from build123d import *

# Parameters (mm, degrees)
ESQUISSE1_R                  = 28
BOSS_EXTRU_1_DEPTH           = 3
ENL_V_MAT_EXTRU_1_DEPTH      = 40.711459303
ENL_V_MAT_EXTRU_1_DEPTH_BACK = 40.711459303
ESQUISSE2_R                  = 3
ESQUISSE3_R                  = 12.75
ESQUISSE3_R_2                = 10.25
BOSS_EXTRU_2_DEPTH           = 10
CHANFREIN1_SIZE              = 2


with BuildPart() as part:
    # Esquisse1 → Boss.-Extru.1 (new body)
    with BuildSketch(Plane.XY):
        Circle(ESQUISSE1_R)
    extrude(amount=BOSS_EXTRU_1_DEPTH)

    # Esquisse2 → Enlèv. mat.-Extru.1 (cut, two sides: drawn at the far end of the back side and taken through both)
    with BuildSketch(Plane.XY.offset(3).offset(-ENL_V_MAT_EXTRU_1_DEPTH_BACK)):
        Circle(ESQUISSE2_R)
    extrude(amount=ENL_V_MAT_EXTRU_1_DEPTH + ENL_V_MAT_EXTRU_1_DEPTH_BACK, mode=Mode.SUBTRACT)

    # Esquisse3 → Boss.-Extru.2 (add)
    with BuildSketch(Plane.XY.offset(3)):
        Circle(ESQUISSE3_R)
        Circle(ESQUISSE3_R_2, mode=Mode.SUBTRACT)
    extrude(amount=BOSS_EXTRU_2_DEPTH)

    # Chanfrein1
    chanfrein1_edges = [part.edges().sort_by_distance(p)[0] for p in [
        (-12.75, 0, 3),
    ]]
    chamfer(chanfrein1_edges, length=CHANFREIN1_SIZE)


solid = part.part
For this review, take the finished solid that the model builds, in its own axes (mm). A direction names the side the tool comes from. Round coordinates to 2 decimals unless told otherwise and drop trailing zeros. Order: outer loops, then holes, each group sorted by start corner. A loop starts at its lowest first (then second) coordinate and runs counter-clockwise, first axis right, second up. Notation, with made-up numbers: (-20.5, -30) -> (-0.5, -30) arc R10 ccw to (-0.5, -19) -> close; hole circle Ø8 at (38.25, -1.5). An arc over 180 degrees is marked (long way). Write item = value, one per line. Start each with the question number.
1) To check wall thickness, follow line 1 (Y direction, x = 0, z = 5.25); line 2 (Z direction, x = 20, y = -1); line 3 (Y direction, x = -5, z = 6). State the ranges of each line that lie inside material, in increasing order. Write a range as from..to.
2) The part is to be moulded in two halves that separate along Y. For faces 1 (the face through (12, -12, 3)), 2 (the face through (-2.764, -12.447, 8.944)), 3 (the face through (-3, 0, 1)), say which applies: +Y half, -Y half, draft (parallel to the pull), parting line (faces both ways), or undercut.
3) Take a section at A-A on x = 0. State the section outline as (y, z) points.
4) Insertion check: pin 1 (4 mm diameter, centred on y = 19, z = 2, fed in from +X); pin 2 (8 mm diameter, centred on x = 6, y = -17.5, fed in from +Z); pin 3 (3 mm diameter, centred on y = 15.5, z = 6, fed in from +X); pin 4 (5 mm diameter, centred on x = -3, z = 11.5, fed in from -Y). Each pin has a flat end and moves straight along its axis. Give the tip position at first contact, or say it passes through.
5) Take a section at C-C on z = 8.25. State the section outline as (x, y) points, plus the area to 3 significant figures.
6) Tool access review of faces 4 (the face through (-2.222, -10.006, 7.93)), 5 (the face through (-9, 6, 13)): name each direction out of +Z, -Z, +X, -X, +Y, -Y from which nothing blocks a thin tool from reaching the whole face with its end or side.
7) Take a section at D-D on y = -16. State the section outline as (x, z) points, plus the area to 3 significant figures.
Verdict:
q1.line_1 = -12.75..-10.25, 10.25..12.75
q1.line_2 = 0..3
q1.line_3 = -11.73..-8.95, 8.95..11.73
q2.face_1 = draft
q2.face_2 = parting line
q2.face_3 = undercut
q3.outline = (-28, 0) -> (-3, 0) -> (-3, 3) -> (-10.25, 3) -> (-10.25, 13) -> (-12.75, 13) -> (-12.75, 5) -> (-14.75, 3) -> (-28, 3) -> close; (3, 0) -> (28, 0) -> (28, 3) -> (14.75, 3) -> (12.75, 5) -> (12.75, 13) -> (10.25, 13) -> (10.25, 3) -> (3, 3) -> close
q4.pin_1 = 22.25
q4.pin_2 = 3.25
q4.pin_3 = through
q4.pin_4 = -12.74
q5.outline = circle Ø25.5 at (0, 0); hole circle Ø20.5 at (0, 0)
q5.area = 181 mm2
q6.face_4 = +Z
q6.face_5 = +Z, +X, -X, +Y, -Y
q7.outline = (-22.98, 0) -> (22.98, 0) -> (22.98, 3) -> (-22.98, 3) -> close
q7.area = 138 mm2
